from build123d import *

# Parameters (mm, degrees)
F1_DEPTH      = 3.75
F1_DEPTH_BACK = 3.75
F2_W          = 3.5
F2_H          = 3.5
F3_DEPTH      = 5.001
F4_R          = 3.74999
F5_R          = 3.74999


# Not quite as in the source:
# - a fillet or chamfer is up to 0.001 mm smaller than in the source, because OpenCascade refuses the exact size


with BuildPart() as f1:
    # F0 (on Front) → F1 (new body, two sides)
    with BuildSketch(Plane.XZ) as f1_sk:
        Polygon((0, 5), (0, 0), (10, 0), (18.0723418804, 8), (68.0723418804, 8), (68.0723418804, 13), (18.0723418804, 13), (10, 5), align=None)
    extrude(amount=F1_DEPTH)
    extrude(f1_sk.sketch, amount=-F1_DEPTH_BACK)

    # F2 (on face) → F3 (cut, through all)
    with BuildSketch(Plane.XY.offset(5)):
        with Locations((3.75, 0)):
            Rectangle(F2_W, F2_H)
    extrude(amount=-F3_DEPTH, mode=Mode.SUBTRACT)

    # F4 (radius 3.75 in the source; OpenCascade refuses exactly that, so slightly less here)
    f4_edges = [f1.edges().sort_by_distance(p)[0] for p in [
        (0, -3.75, 2.5),
        (0, 3.75, 2.5),
    ]]
    fillet(f4_edges, radius=F4_R)

    # F5 (radius 3.75 in the source; OpenCascade refuses exactly that, so slightly less here)
    f5_edges = [f1.edges().sort_by_distance(p)[0] for p in [
        (68.072342, -3.75, 10.5),
        (68.072342, 3.75, 10.5),
    ]]
    fillet(f5_edges, radius=F5_R)


solid = f1.part
Source: CAD feature listing. Evaluate the final solid. Frame: model axes, mm. A direction names the side the tool comes from. Coordinates: 2 decimals unless noted, no trailing zeros. Loops run counter-clockwise (first coordinate to the right, second up) from the corner with the lowest first, then second, coordinate; pieces in that order, holes last. Notation, with made-up numbers: (8, 66) - (65, 66) arc R12 cw to (65, 75) - close; hole circle Ø8 at (-13.5, 88). An arc over 180 degrees is marked (long way). One line per question, with ' | ' between items.
1) Section A-A, the plane y = 1. Return loops of the section in (x, z), then the cut area to 3 significant figures.
Report:
outline: (0.14, 0) - (2, 0) - (2, 5) - (0.14, 5) - close; (5.5, 0) - (10, 0) - (18.07, 8) - (67.94, 8) - (67.94, 13) - (18.07, 13) - (10, 5) - (5.5, 5) - close | area: 322 mm²
2) Set-up query: faces 1 (the face through (5.5, 0, 3)), 2 (the face through (6, 0, 5)), 3 (the face through (66.945, -2.681, 10.535)). Return all of +Z, -Z, +X, -X, +Y, -Y with unobstructed straight access to the full face (end or side cutting, diameter ignored); none if empty.
Report:
face 1: +Z, -Z | face 2: +Z, -X, +Y, -Y | face 3: +Z, -Z, +X, -Y
3) Section C-C, the plane x = 43. Return loops of the section in (y, z), then the cut area to 3 significant figures.
Report:
outline: (-3.75, 8) - (3.75, 8) - (3.75, 13) - (-3.75, 13) - close | area: 37.5 mm²
4) Line query: line 1 along Z through (x, y) = (31.5, 3); line 2 along X through (y, z) = (-0.75, 3); line 3 along X through (y, z) = (-2.75, 8.75). Output: solid intervals per line, ascending.
Report:
line 1: z = 8 to 13 | line 2: x = 0.08 to 2, 5.5 to 13.03 | line 3: x = 13.78 to 66.87
5) Pull-direction query (Y, two-part tool) for faces 4 (the face through (43, 0, 8)), 5 (the face through (1.069, 2.622, 2.465)), 6 (the face through (4, 1.75, 3)), 7 (the face through (1.069, -2.622, 2.465)); classes: released by +Y, released by -Y, zero draft, split by the parting line, or undercut.
Report:
face 4: zero draft | face 5: released by +Y | face 6: undercut | face 7: released by -Y
6) First-contact query: P1, Ø1, axis at y = 2.5, z = 10.5, coming from the +X side; P2, Ø1.5, axis at y = -0.5, z = 2.5, coming from the +X side; P3, Ø2, axis at x = 26.5, y = 0, coming from the -Z side. Flat tips, straight axial feed; report the tip coordinate or a pass-through.
Report:
P1: stops at x = 67.49 | P2: stops at x = 13.28 | P3: stops at z = 8
